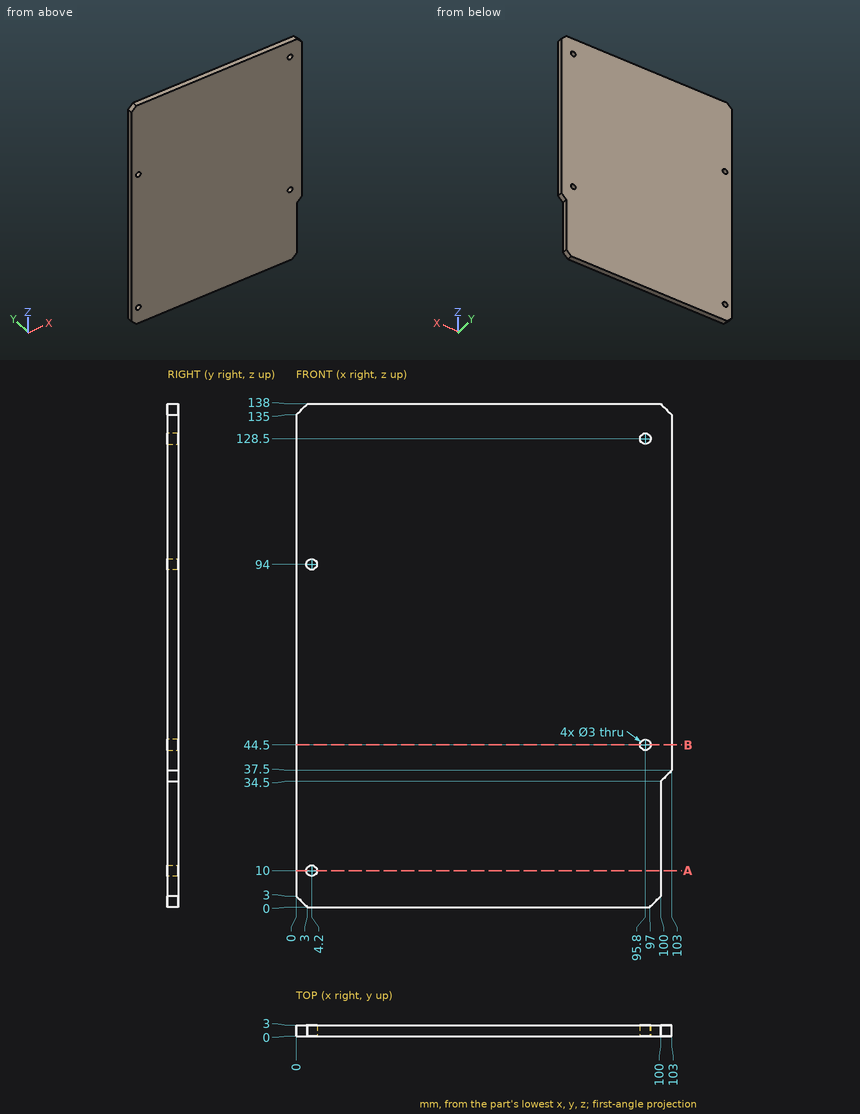
Print and shaded views of the part. All mm, measured from the part's lowest x, y and z. Coordinates: 2 decimals unless noted, no trailing zeros. Loops run counter-clockwise (first coordinate to the right, second up) from the corner with the lowest first, then second, coordinate; pieces in that order, holes last. Notation, with made-up numbers: (-15, 56) -> (39, 56) arc R26 ccw to (39, 81) -> close; hole circle Ø4 at (57, 79). An arc over 180 degrees is marked (long way). Use a Markdown table: item, result. Add a question column.
Item 1: Band-saw the part on A-A on z = 10. Write the cut outline in (x, y), plus the area to 3 significant figures.
Item 2: Flat gauge pins, fed straight in: P1, Ø1.5, axis at y = 1, z = 24, coming from the +X side; P2, Ø1.8, axis at x = 4.2, z = 94, coming from the -Y side. Where does each tip first touch, or does it go through?
Item 3: Band-saw the part on B-B on z = 44.5. Write the cut outline in (x, y), plus the area to 3 significant figures.
Item 4: Probe probe 1 along Z at (x, y) = (95.8, 1.5); probe 2 along X at (y, z) = (0.65, 128.5); probe 3 along X at (y, z) = (0.8, 94). List the from-to ranges inside material, lowest first.
Geometry says:
| question | item | result |
|---|---|---|
| 1 | outline | (0, 0) -> (2.7, 0) -> (2.7, 3) -> (0, 3) -> close; (5.7, 0) -> (100, 0) -> (100, 3) -> (5.7, 3) -> close |
| 1 | area | 291 mm² |
| 2 | P1 | x = 100 |
| 2 | P2 | through |
| 3 | outline | (0, 0) -> (94.3, 0) -> (94.3, 3) -> (0, 3) -> close; (97.3, 0) -> (103, 0) -> (103, 3) -> (97.3, 3) -> close |
| 3 | area | 300 mm² |
| 4 | probe 1 | 0 to 43, 46 to 127, 130 to 138 |
| 4 | probe 2 | 0 to 94.3, 97.3 to 103 |
| 4 | probe 3 | 0 to 2.7, 5.7 to 103 |
